Check sheet for the modelled part. Datum: model origin and axes. Units: mm. A direction names the side the tool comes from. Round coordinates to 2 decimals unless told otherwise and drop trailing zeros. Order: outer loops, then holes, each group sorted by start corner. A loop starts at its lowest first (then second) coordinate and runs counter-clockwise, first axis right, second up.
(1) Mould release check, pull along Z, two halves, no side actions. Record for faces 1 (the cylindrical face through (45.332, -16.919, 17.798)), 2 (the cylindrical face through (-7.559, -3.131, -5.796)), 3 (the flat face through (20, -20, 16.51)), 4 (the cylindrical face through (-0.33, -17.8, 14.44)): released by +Z, released by -Z, zero draft, split by the parting line, or undercut.
(2) Depth check by flat-ended pin: pin 1 (12 mm diameter, centred on y = -6, z = -13.5, fed in from -X); pin 2 (4 mm diameter, centred on y = -5, z = -6.5, fed in from +X); pin 3 (3 mm diameter, centred on y = -20.5, z = 18, fed in from -X). Enter the tip coordinate at first touch or a pass-through.
(3) Tool access check on faces 5 (the flat face through (-5.08, -20, 18)), 6 (the flat face through (20, -24.13, 18)), 7 (the flat face through (21, -16.51, 18)). Record the directions out of +Z, -Z, +X, -X, +Y, -Y that give a thin tool (end or side, any length) a straight path to the whole face; none if there is none.
(4) Sectioned sample at D-D, the plane y = -4.5. Enter the section's corners in (x, z) (3 decimals), and give its area (3 significant figures).
(5) Sectioned sample at A-A, the plane z = -5. Enter the section's corners in (x, y), and give its area (3 significant figures).
(6) Sectioned sample at C-C, the plane x = 16. Enter the section's corners in (y, z).
(7) Sectioned sample at B-B, the plane y = -20.32. Enter the section's corners in (x, z), and give its area (3 significant figures).
(8) Thickness scan on probe 1 along X at (y, z) = (-27, 0); probe 2 along Z at (x, y) = (-7, -22); probe 3 along Y at (x, z) = (-1.5, -4.5). Record the ranges inside material, lowest first.
```python
from build123d import *

# Parameters (mm, degrees)
F0_R      = 9.525
F1_DEPTH  = 6.35
F2_R      = 12.7
F3_DEPTH  = 25.4
F6_R      = 12.7
F7_DEPTH  = 19.05
F8_R      = 2.54
F9_DEPTH  = 19.05
F10_R     = 2.54
F11_DEPTH = 2.54


with BuildPart() as f1:
    # F0 (on Front) → F1 (new body)
    with BuildSketch(Plane.XZ):
        Circle(F0_R)
    extrude(amount=F1_DEPTH)

    # F2 (on face) → F3 (join)
    with BuildSketch(Plane.XZ.offset(6.35)):
        Circle(F2_R)
    extrude(amount=F3_DEPTH)

    # F4 (on Right) → F5 (revolve)
    with BuildSketch(Plane.YZ):
        with BuildLine():
            Line((-31.75, 0), (-31.75, 12.7))
            ThreePointArc((-31.75, 12.7), (-40.730256, 8.980256), (-44.45, 0))
            Line((-44.45, 0), (-31.75, 0))
        make_face()
    revolve(axis=Axis((0, -31.75, 6.35), (0, 0, 1)))

    # F6 (on face) → F7 (join)
    with BuildSketch(Plane(origin=(0, 0, 0), x_dir=(1, 0, 0), z_dir=(0, 0, -1))):
        with Locations((0, 31.75)):
            Circle(F6_R)
    extrude(amount=F7_DEPTH)

    # F8 (on Top) → F9 (join)
    with BuildSketch(Plane.XY):
        with Locations((0, -20.32)):
            Circle(F8_R)
    extrude(amount=F9_DEPTH)

    # F10 (on face) → F11 (join)
    with BuildSketch(Plane.XY.offset(19.05)):
        with BuildLine():
            ThreePointArc((45.72, -17.869775), (45.321731, -16.908269), (44.360225, -16.51))
            Line((44.360225, -16.51), (-3.720225, -16.51))
            ThreePointArc((-3.720225, -16.51), (-4.681731, -16.908269), (-5.08, -17.869775))
            Line((-5.08, -17.869775), (-5.08, -22.770225))
            ThreePointArc((-5.08, -22.770225), (-4.681731, -23.731731), (-3.720225, -24.13))
            Line((-3.720225, -24.13), (44.360225, -24.13))
            ThreePointArc((44.360225, -24.13), (45.321731, -23.731731), (45.72, -22.770225))
            Line((45.72, -22.770225), (45.72, -17.869775))
        make_face()
        with Locations((0, -20.32)):
            Circle(F10_R, mode=Mode.SUBTRACT)
    extrude(amount=-F11_DEPTH)


solid = f1.part
```
Derived:
1. face 1: zero draft
1. face 2: split by the parting line
1. face 3: undercut
1. face 4: undercut
2. pin 1: stops at x = -10.24
2. pin 2: stops at x = 11.66
2. pin 3: stops at x = -5.08
3. face 5: +Z, -X, +Y, -Y
3. face 6: +Z, +X, -X, -Y
3. face 7: +Z, +X, -X, +Y
4. outline: circle Ø19.05 at (0, 0)
4. area: 285 mm2
5. outline: (-11.67, -26.75) arc R12.7 ccw (long way) to (11.67, -26.75) - (11.67, -6.35) - (8.11, -6.35) - (8.11, 0) - (-8.11, 0) - (-8.11, -6.35) - (-11.67, -6.35) - close
5. area: 956 mm2
6. outline: (-24.13, 16.51) - (-16.51, 16.51) - (-16.51, 19.05) - (-24.13, 19.05) - close
7. outline: (-5.54, -19.05) - (5.54, -19.05) - (5.54, -11.43) arc R12.7 ccw to (2.54, 12.44) - (2.54, 16.51) - (45.72, 16.51) - (45.72, 19.05) - (-5.08, 19.05) - (-5.08, 16.51) - (-2.54, 16.51) - (-2.54, 12.44) arc R12.7 ccw to (-5.54, -11.43) - close
7. area: 730 mm2
8. probe 1: x = -12.7 to 12.7
8. probe 2: z = -19.05 to 10.6
8. probe 3: y = -44.36 to 0
